Build history of the part. All positions in model axes, mm. Round coordinates to 2 decimals unless told otherwise and drop trailing zeros. Write each loop counter-clockwise with the first axis right and the second up, starting at its lowest first coordinate (ties: lowest second). Pieces come first, ordered by that corner, then holes. Notation, with made-up numbers: M 22.5,-4 L 36.5,-4 A22 cw 36.5,15 Z; hole C 15,42 d9. An arc over 180 degrees is marked long. Write item = value, one per line. Start each with the question number.
Q1. Probe L1, parallel to Y at x = 12.5, z = 0.4; L2, parallel to Y at x = 10, z = 2.85 (3 decimals); L3, parallel to X at y = 60, z = 1.6. List the from-to ranges inside material, lowest first.
Q2. Band-saw the part on C-C on y = 60.5. Write the cut outline in (x, z) (3 decimals).
Q3. Band-saw the part on A-A on z = 1.4. Write the cut outline in (x, y) (1 decimal).
Q4. Drop flat-ended pins along their axis: P1, Ø0.8, axis at x = -0.5, z = 1.5, coming from the -Y side (3 decimals); P2, Ø1, axis at y = 3.5, z = 1, coming from the +X side (3 decimals). Give the stop position or say it passes through.
Q5. Band-saw the part on B-B on x = 20. Write the cut outline in (y, z) (3 decimals).
```python
from build123d import *

# Parameters (mm, degrees)
BOSS_EXTRUDE1_DEPTH = 3.175


with BuildPart() as part:
    # Sketch1 → Boss-Extrude1 (new body)
    with BuildSketch(Plane.XY):
        with BuildLine():
            Line((9.525, 9.525), (11.1125, 9.525))
            ThreePointArc((11.1125, 9.525), (20.092756121, 13.244743879), (23.8125, 22.225))
            Line((23.8125, 22.225), (23.8125, 50.8))
            ThreePointArc((23.8125, 50.8), (20.092756121, 59.780256121), (11.1125, 63.5))
            Line((11.1125, 63.5), (-1.5875, 63.5))
            ThreePointArc((-1.5875, 63.5), (-10.567756121, 59.780256121), (-14.2875, 50.8))
            Line((-14.2875, 50.8), (-14.2875, 22.225))
            ThreePointArc((-14.2875, 22.225), (-10.567756121, 13.244743879), (-1.5875, 9.525))
            Line((-1.5875, 9.525), (0, 9.525))
            Line((0, 9.525), (0, 0))
            Line((0, 0), (9.525, 0))
            Line((9.525, 0), (9.525, 9.525))
        make_face()
    extrude(amount=BOSS_EXTRUDE1_DEPTH)


solid = part.part
```
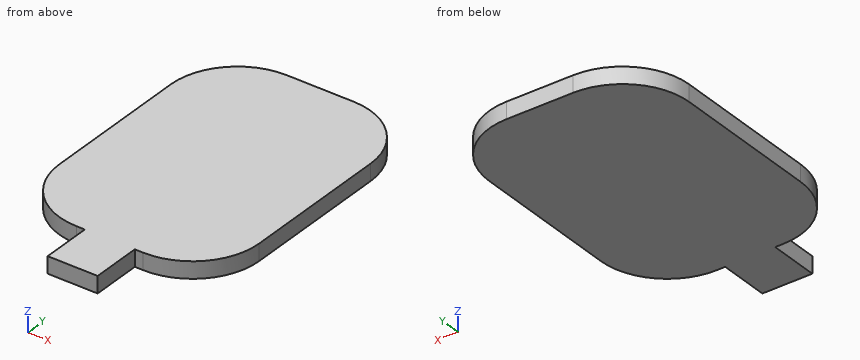
Conclusion:
q1.L1 = 9.6 to 63.42
q1.L2 = 9.525 to 63.5
q1.L3 = -10.34 to 19.87
q2.outline = M -9.785,0 L 19.31,0 L 19.31,3.175 L -9.785,3.175 Z
q3.outline = M -14.3,22.2 A12.7 ccw -1.6,9.5 L 0,9.5 L 0,0 L 9.5,0 L 9.5,9.5 L 11.1,9.5 A12.7 ccw 23.8,22.2 L 23.8,50.8 A12.7 ccw 11.1,63.5 L -1.6,63.5 A12.7 ccw -14.3,50.8 Z
q4.P1 = 9.525
q4.P2 = 9.525
q5.outline = M 13.153,0 L 59.872,0 L 59.872,3.175 L 13.153,3.175 Z
